```python
from build123d import *

# Parameters (mm, degrees)
SKETCH_1_R      = 3
EXTRUDE_1_DEPTH = 10


with BuildPart() as part:
    # 草图1 → 凸台-拉伸1 (new body)
    with BuildSketch(Plane(origin=(0, 0, 0), x_dir=(1, 0, 0), z_dir=(0, 1, 0))):
        with BuildLine():
            Line((-50, 0), (0, 0))
            Line((0, 0), (50, 0))
            ThreePointArc((50, 0), (35.355339059, 35.355339059), (0, 50))
            ThreePointArc((0, 50), (-10, 40), (0, 30))
            ThreePointArc((0, 30), (15, 25.980762114), (25.980762114, 15))
            Line((25.980762114, 15), (-30, 15))
            Line((-30, 15), (-30, 30))
            Line((-30, 30), (-50, 30))
            Line((-50, 30), (-50, 0))
        make_face()
        with Locations(Location((0, 40, 0), (0, 0, 270))):
            Circle(SKETCH_1_R, mode=Mode.SUBTRACT)
    extrude(amount=EXTRUDE_1_DEPTH)


solid = part.part
```
Model file for the job. Use its own axes, mm. A direction names the side the tool comes from. Coordinates: 2 decimals unless noted, no trailing zeros. Loops run counter-clockwise (first coordinate to the right, second up) from the corner with the lowest first, then second, coordinate; pieces in that order, holes last. Notation, with made-up numbers: (14.5, 22) - (27.5, 22) arc R18 ccw to (27.5, 49) - close; hole circle Ø4 at (-22.75, 67). An arc over 180 degrees is marked (long way). Write item = value, one per line. Start each with the question number.
Item 1: 3-axis set-ups, long thin cutter, end or side, ignore diameter. For faces 5 (the face through (-40, 5, -30)), 6 (the face through (-2, 5, -15)), 7 (the face through (-30, 5, -22)): which of +Z, -Z, +X, -X, +Y, -Y reach the whole face in a straight line?
Item 2: Wall check: probe 1 along Z at (x, y) = (-2, 2.75); probe 2 along Z at (x, y) = (-2.5, 2.25); probe 3 along X at (y, z) = (7, -40). Give the ranges that are in metal, low to high. Write a range as [from, to].
Item 3: Saw through at B-B, the plane z = -40. List the corners of the cut face in (x, y).
Item 4: Saw through at A-A, the plane x = -6. List the corners of the cut face in (y, z).
Item 5: Drop flat-ended pins along their axis: pin 1 Ø4 at (y, z) = (8, -42.5) entering from -X; pin 2 Ø5 at (y, z) = (2, -15) entering from +X; pin 3 Ø4 at (x, y) = (-7.5, 9) entering from -Z. Give the stop position or say it passes through.
Item 6: Saw through at C-C, the plane y = 6. List the corners of the cut face in (x, z), then the cut area to 3 significant figures.
Item 7: Saw through at D-D, the plane x = -37. List the corners of the cut face in (y, z), then the cut area to 3 significant figures.
Item 8: Pull direction Z, two halves, no side cores. Call faces 1 (the face through (-1, 0, -14)), 2 (the face through (35.742, 4.93, -34.964)), 3 (the face through (14.81, 4.93, -26.09)), 4 (the face through (0, 5, -43)): +Z half, -Z half, draft (parallel to the pull), parting line (faces both ways), or undercut.
Answers:
q1.face_5 = -Z, -X, +Y, -Y
q1.face_6 = +Y, -Y
q1.face_7 = -Z, +Y, -Y
q2.probe_1 = [-49.8, -42.24], [-37.76, -30.2], [-15, 0]
q2.probe_2 = [-49.68, -41.66], [-38.34, -30.32], [-15, 0]
q2.probe_3 = [-10, -3], [3, 30]
q3.outline = (-10, 0) - (-3, 0) - (-3, 10) - (-10, 10) - close; (3, 0) - (30, 0) - (30, 10) - (3, 10) - close
q4.outline = (0, -48) - (10, -48) - (10, -32) - (0, -32) - close; (0, -15) - (10, -15) - (10, 0) - (0, 0) - close
q5.pin_1 = -9.99
q5.pin_2 = 48.41
q5.pin_3 = -48.35
q6.outline = (-50, -30) - (-30, -30) - (-30, -15) - (25.98, -15) arc R30 cw to (0, -30) arc R10 ccw to (0, -50) arc R50 ccw to (50, 0) - (-50, 0) - close; hole circle Ø6 at (0, -40)
q6.area = 2,870 mm2
q7.outline = (0, -30) - (10, -30) - (10, 0) - (0, 0) - close
q7.area = 300 mm2
q8.face_1 = draft
q8.face_2 = -Z half
q8.face_3 = undercut
q8.face_4 = undercut
